from build123d import *

# Parameters (mm, degrees)
SKETCH1_R           = 1.1
SKETCH1_W           = 23.2
SKETCH1_H           = 12.2
SKETCH1_R_2         = 2
BOSS_EXTRUDE1_DEPTH = 3.175
CHAMFER1_SIZE       = 15


with BuildPart() as part:
    # Sketch1 → Boss-Extrude1 (new body)
    # profile 1 of 3: a face of its own
    with BuildSketch(Plane.XY):
        Polygon((10.8, 21.8), (10.8, 34), (3.175, 34), (3.175, 26), (0, 26), (0, 19.9), (3.175, 19.9), (3.175, 17), (40, 17), (40, 34), (34, 34), (34, 21.8), align=None)
        with Locations((8.65, 27.9)):
            Circle(SKETCH1_R, mode=Mode.SUBTRACT)
        with Locations((36.15, 27.9)):
            Circle(SKETCH1_R, mode=Mode.SUBTRACT)
    # profile 2 of 3: a face of its own
    with BuildSketch(Plane.XY):
        Polygon((40, 0), (40, 17), (3.175, 17), (3.175, 15), (8.5, 15), (8.5, 16.625), (12, 16.625), (12, 15), (20, 15), (20, 11), (12, 11), (12, 9.375), (8.5, 9.375), (8.5, 11), (3.175, 11), (3.175, 6.1), (0, 6.1), (0, 0), align=None)
    # profile 3 of 3: a face of its own
    with BuildSketch(Plane.XY):
        with Locations((22.4, 27.9)):
            Rectangle(SKETCH1_W, SKETCH1_H)
        with Locations((16.9, 27.9)):
            Circle(SKETCH1_R_2, mode=Mode.SUBTRACT)
    extrude(amount=BOSS_EXTRUDE1_DEPTH)

    # Chamfer1
    chamfer1_edges = [part.edges().sort_by_distance(p)[0] for p in [
        (40, 0, 1.5875),
    ]]
    chamfer(chamfer1_edges, length=CHAMFER1_SIZE)


solid = part.part
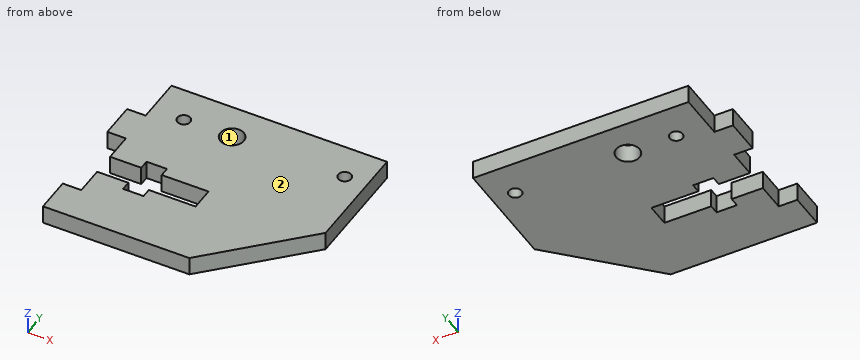
Geometry check sheet. Reference: the model listing, model coordinates, mm. Face numbers are marked on the shaded views. Coordinates: 2 decimals unless noted, no trailing zeros. Order: outer loops, then holes, each group sorted by start corner. A loop starts at its lowest first (then second) coordinate and runs counter-clockwise, first axis right, second up. Notation, with made-up numbers: (88.5, 49) -> (98.5, 49) arc R13 cw to (98.5, 66) -> close; hole circle Ø1 at (79.25, 13). An arc over 180 degrees is marked (long way). Use a Markdown table: item, result. Add a question column.
1. Cross-section at D-D (x = 36.15). Enter the section's corners in (y, z) (3 decimals), and give its area (3 significant figures).
2. Cross-section at C-C (z = 1.25). Enter the section's corners in (x, y) (3 decimals), and give its area (3 significant figures).
3. Go/stop test with flat-tipped pins: pin 1 Ø1 at (y, z) = (31.5, 1.5) entering from -X (3 decimals); pin 2 Ø1.8 at (y, z) = (10, 1) entering from +X. Record where each tip stops, or that it passes through.
4. Material ranges on L1, parallel to Y at x = 8.65, z = 1.4 (3 decimals); L2, parallel to Y at x = 16.9, z = 0.85; L3, parallel to X at y = 16.5, z = 2.4 (3 decimals), recorded low to high.
5. Cross-section at A-A (y = 27.9). Enter the section's corners in (x, z) (3 decimals).
6. Mould release check, pull along X, two halves, no side actions. Record for the marked faces 1 and 2: pulls with the +X half, pulls with the -X half, needs draft (parallel to the pull), parting line crosses it, or undercut.
7. Cross-section at B-B (x = 16.9). Enter the section's corners in (y, z) (3 decimals), and give its area (4 significant figures).
Filled sheet:
| question | item | result |
|---|---|---|
| 1 | outline | (11.15, 0) -> (26.8, 0) -> (26.8, 3.175) -> (11.15, 3.175) -> close; (29, 0) -> (34, 0) -> (34, 3.175) -> (29, 3.175) -> close |
| 1 | area | 65.6 mm2 |
| 2 | outline | (0, 0) -> (25, 0) -> (40, 15) -> (40, 34) -> (3.175, 34) -> (3.175, 26) -> (0, 26) -> (0, 19.9) -> (3.175, 19.9) -> (3.175, 15) -> (8.5, 15) -> (8.5, 16.625) -> (12, 16.625) -> (12, 15) -> (20, 15) -> (20, 11) -> (12, 11) -> (12, 9.375) -> (8.5, 9.375) -> (8.5, 11) -> (3.175, 11) -> (3.175, 6.1) -> (0, 6.1) -> close; hole circle Ø2.2 at (8.65, 27.9); hole circle Ø4 at (16.9, 27.9); hole circle Ø2.2 at (36.15, 27.9) |
| 2 | area | 1,080 mm2 |
| 3 | pin 1 | x = 3.175 |
| 3 | pin 2 | x = 35.9 |
| 4 | L1 | 0 to 9.375, 16.625 to 26.8, 29 to 34 |
| 4 | L2 | 0 to 11, 15 to 25.9, 29.9 to 34 |
| 4 | L3 | 3.175 to 8.5, 12 to 40 |
| 5 | outline | (3.175, 0) -> (7.55, 0) -> (7.55, 3.175) -> (3.175, 3.175) -> close; (9.75, 0) -> (14.9, 0) -> (14.9, 3.175) -> (9.75, 3.175) -> close; (18.9, 0) -> (35.05, 0) -> (35.05, 3.175) -> (18.9, 3.175) -> close; (37.25, 0) -> (40, 0) -> (40, 3.175) -> (37.25, 3.175) -> close |
| 6 | face 1 | undercut |
| 6 | face 2 | needs draft |
| 7 | outline | (0, 0) -> (11, 0) -> (11, 3.175) -> (0, 3.175) -> close; (15, 0) -> (25.9, 0) -> (25.9, 3.175) -> (15, 3.175) -> close; (29.9, 0) -> (34, 0) -> (34, 3.175) -> (29.9, 3.175) -> close |
| 7 | area | 82.55 mm2 |
